Could you check a few things on this model? Use its own coordinates, in mm. A direction names the side the tool comes from. Give positions to 0.01 mm unless a question says otherwise; leave off trailing zeros. Order: outer loops, then holes, each group sorted by start corner. A loop starts at its lowest first (then second) coordinate and runs counter-clockwise, first axis right, second up. Notation, with made-up numbers: M 64.5,70 L 121.5,70 A29 cw 121.5,109 Z; hole C 79.5,40 d3. An arc over 180 degrees is marked long. Use a Markdown table: item, result. Add a question column.
Solid Edge part; units mm, degrees
sketch "Sketch1" plane through (0, 0, 0) normal (0, 0, 1) x (1, 0, 0)
  circle A0 centre (0, 0) radius 6
  circle A1 centre (0, 0) radius 2
extrude "Protrusion1" add sketch "Sketch1" along normal blind 5
sketch "Sketch2" plane through (0, 0, 0) normal (0, 0, -1) x (0, 1, 0)
  line L0 (4, 4.4721) -> (-4, 4.4721)
  line L1 (-4, 4.4721) -> (-4, 30)
  line L2 (-4, 30) -> (4, 30)
  line L3 (4, 30) -> (4, 4.4721)
  dimension "D1" = 4
extrude "ExtrudedProtrusion_2" add sketch "Sketch2" against normal blind 3
sketch "Sketch3" plane through (14.7361, 0, 3) normal (0, 0, 1) x (1, 0, 0)
  line L0 (15.2639, 4) -> (7.2639, 4)
  line L1 (7.2639, 4) -> (7.2639, -4)
  line L2 (7.2639, -4) -> (15.2639, -4)
  line L3 (15.2639, -4) -> (15.2639, 4)
  dimension "D1" = 15.2639
extrude "ExtrudedProtrusion_3" add sketch "Sketch3" along normal blind 5
properties material "Polyethylene, low density"
1) For faces 4 (the face through (20, 4, 2)), 5 (the face through (3, 0, 5)), 6 (the face through (22, 0, 5)), which set-ups out of +Z, -Z, +X, -X, +Y, -Y let a thin tool reach every point of the face, with its end or its side?
2) Suppose I cut it at C-C on z = 1.5. Please give me the cut outline in (x, y), and give its area (3 significant figures).
3) For pin 1 (1.5 mm diameter, centred on x = -1.5, y = 0, fed in from +Z); pin 2 (2.5 mm diameter, centred on x = 20.5, z = 2, fed in from -Y), each with a flat end and sliding along its axis, tell me the tip position at first contact or that it passes through.
4) Suppose I cut it at D-D on y = 3.5. Please give me the cut outline in (x, z), and give its area (3 significant figures).
5) Please list where these lines run through material, in increasing order: line 1 (Y direction, x = 0, z = 2.5); line 2 (Z direction, x = 19.5, y = 3.5); line 3 (Y direction, x = 28, z = 1). Write a range as from..to.
6) We'd pull the mould along X, two halves only. Please class faces 1 (the face through (13, 0, 3)), 2 (the face through (30, 0, 4)), 3 (the face through (20, -4, 2)): pulls with the +X half, pulls with the -X half, needs draft (parallel to the pull), parting line crosses it, or undercut.
7) Suppose I cut it at A-A on x = 0. Please give me the cut outline in (y, z), and give its area (3 significant figures).
8) Suppose I cut it at B-B on y = 0. Please give me the cut outline in (x, z), and give its area (3 significant figures).
Values found:
| question | item | result |
|---|---|---|
| 1 | face 4 | +Z, -Z, +X, +Y |
| 1 | face 5 | +Z, -X, +Y, -Y |
| 1 | face 6 | +Z, +Y, -Y |
| 2 | outline | M 4.47,-4 L 30,-4 L 30,4 L 4.47,4 A6 ccw long Z; hole C 0,0 d4 |
| 2 | area | 296 mm^2 |
| 3 | pin 1 | stops at z = 5 |
| 3 | pin 2 | stops at y = -4 |
| 4 | outline | M -4.87,0 L 30,0 L 30,8 L 22,8 L 22,3 L 4.87,3 L 4.87,5 L -4.87,5 Z |
| 4 | area | 164 mm^2 |
| 5 | line 1 | y = -6..-2, 2..6 |
| 5 | line 2 | z = 0..3 |
| 5 | line 3 | y = -4..4 |
| 6 | face 1 | undercut |
| 6 | face 2 | pulls with the +X half |
| 6 | face 3 | needs draft |
| 7 | outline | M -6,0 L -2,0 L -2,5 L -6,5 Z; M 2,0 L 6,0 L 6,5 L 2,5 Z |
| 7 | area | 40.0 mm^2 |
| 8 | outline | M -6,0 L -2,0 L -2,5 L -6,5 Z; M 2,0 L 30,0 L 30,8 L 22,8 L 22,3 L 6,3 L 6,5 L 2,5 Z |
| 8 | area | 152 mm^2 |
